Verification items for the finished model (mm, model axes). A direction names the side the tool comes from. Give positions to 0.01 mm unless a question says otherwise; leave off trailing zeros. Write each loop counter-clockwise with the first axis right and the second up, starting at its lowest first coordinate (ties: lowest second). Pieces come first, ordered by that corner, then holes. Notation, with made-up numbers: (2, 7) - (52, 7) arc R35 ccw to (52, 45) - close; hole circle Ø3 at (-22, 46.25). An arc over 180 degrees is marked (long way). Answer as a JSON object with one key per item and string values. Group by question number.
Item 1: Tool access check on faces 1 (the face through (-4.72, 3.48, -1.97)), 2 (the face through (-4.724, -3.448, -2.028)), 3 (the face through (-4.72, -3.48, 1.97)), 4 (the face through (0, 2.5, 2.5)), 5 (the face through (-4.724, 3.448, 2.028)). Record the directions out of +Z, -Z, +X, -X, +Y, -Y that give a thin tool (end or side, any length) a straight path to the whole face; none if there is none.
Item 2: Sectioned sample at A-A, the plane y = 0. Record the boundary of the cut face in (x, z).
Item 3: Scan lines: line 1 along X through (y, z) = (3.25, 1.5); line 2 along X through (y, z) = (-5, 2.5); line 3 along Y through (x, z) = (21, 2.5). Record each from-to range of solid material in increasing order. Write a range as [from, to].
Item 4: Go/stop test with flat-tipped pins: pin 1 (3 mm diameter, centred on x = 10, y = -3, fed in from +Z); pin 2 (5.5 mm diameter, centred on y = -0.5, z = -2.5, fed in from +X); pin 3 (1.5 mm diameter, centred on x = 17, z = 3, fed in from -Y); pin 4 (1.9 mm diameter, centred on x = -5.5, y = 0.5, fed in from -Z). Record where each tip stops, or that it passes through.
Item 5: Sectioned sample at B-B, the plane x = 29.5. Record the boundary of the cut face in (y, z).
Autodesk Inventor part; units mm, degrees
ref_plane "Work Plane1" through (10.95, 0, 0) normal (0, 0, -1) x (1, 0, 0)
ref_plane "YZ Plane" through (0, 0, 0) normal (1, 0, 0) x (0, 1, 0)
ref_plane "XZ Plane" through (0, 0, 0) normal (0, 1, 0) x (-1, 0, 0)
sketch "Schizzo1" plane through (0, 0, 0) normal (0, 0, 1) x (1, 0, 0)
  line L0 (-3.06, 0) -> (-3.06, 4.0996)
  line L1 (0, 5.7) -> (0, 3)
  line L2 (17, 3) -> (35, 3)
  line L3 (35, 3) -> (35, 0)
  line L4 (35, 0) -> (-3.06, 0)
  arc A0 (0, 5.7) -> (-2.0969, 6.1649) centre (-1.1, 5.7) ccw
  line L5 (0, -1.4013) -> (0, 8.4076)
  line L6 (-10.672, 0) -> (42.612, 0)
  line L7 (0, 3) -> (0.0001, 3)
  line L8 (0.0001, 3) -> (0.0001, 3)
  line L9 (0.0001, 3) -> (16.3865, 3)
  line L10 (16.3865, 3) -> (17, 3)
  line L11 (-3.06, 4.0996) -> (-2.0969, 6.1649)
  line L12 (0.0001, 3) -> (17, 3) construction
  line L13 (17, 3) -> (17, 0) construction
  dimension "d0" = 1.1
  dimension "d1" = 35
  dimension "d2" = 18
  dimension "d3" = 13.6
  dimension "d4" = 6
  dimension "d5" = 3.06
  dimension "d15" = 6
  dimension "d16" = 6
  dimension "d17" = 0.0001
  dimension "d18" = 0.6135
  dimension "d19" = 25
revolve "Corpo" add sketch "Schizzo1" angle 360 about axis through (35, 0, 0) along (-1, 0, 0)
sketch "Schizzo2" plane through (0, 0, 0) normal (1, 0, 0) x (0, 0, -1)
  line L0 (4, 2.3094) -> (4, -2.3094)
  line L1 (4, -2.3094) -> (0, -4.6188)
  line L2 (0, -4.6188) -> (-4, -2.3094)
  line L3 (-4, -2.3094) -> (-4, 2.3094)
  line L4 (-4, 2.3094) -> (0, 4.6188)
  line L5 (0, 4.6188) -> (4, 2.3094)
  point P0 (0, 0)
  point P1 (0, 0)
  dimension "d23" = 8
extrude "Testa" add sketch "Schizzo2" against normal blind 6.8
sketch "Schizzo3" plane through (0, 0, 0) normal (0, 0, 1) x (1, 0, 0)
  line L0 (-6.8, 3.8) -> (-6.8, 4.6188)
  line L1 (-6.8, 4.6188) -> (-6.3273, 4.6188)
  line L2 (-6.3273, 4.6188) -> (-6.8, 3.8)
  line L3 (-7.5964, 0) -> (-2.0215, 0)
  line L4 (-6.8, 4.6188) -> (-6.8, 2.3094)
  line L5 (-2.8179, 4.6188) -> (-6.8, 4.6188)
  point P0 (-6.8, 2.3094)
  dimension "d8" = 30
  dimension "d22" = 7.6
revolve "Smusso1" cut sketch "Schizzo3" angle 360 about axis through (-10, 0, 0) along (1, 0, 0)
thread "Filettatura"
chamfer "Smusso2" distance 0.6135 distance2 0.6135 1 edges at (35, -3, 0) measured on face at (35, -0.3546, -0.3912)
ref_plane "Work Plane1" through (10.95, 0, 0) normal (0, 0, -1) x (1, 0, 0)
equation "\"d0\" = PHH"
equation "\"d1\" = NLG"
equation "\"d2\" = GEL"
equation "\"d3\" = LADI"
equation "\"d4\" = GD"
equation "\"d5\" = 0.45 * KOH"
equation "\"d15\" = SD2"
equation "\"d16\" = BDM"
equation "\"d18\" = GAL"
equation "\"d19\" = KEWI"
equation "\"d23\" = SW"
equation "\"d6\" = KOH"
equation "\"d8\" = ANG1"
equation "\"d22\" = SW0"
equation "\"d10\" = GEL"
equation "\"d13\" = -0.5 * SPD + 0.5 * GD"
equation "\"d14\" = GUL"
equation "\"NLG\" = 35"
equation "\"GD\" = NND"
equation "\"BDM\" = NND"
equation "\"KOH\" = 6.8"
equation "\"GEL\" = 18"
equation "\"LADI\" = 13.6"
equation "\"SW\" = 8"
equation "\"PHH\" = RR"
equation "\"SW0\" = 7.6"
equation "\"SPD\" = NND - 1.2269 * PTC"
equation "\"SD2\" = NND"
equation "\"SD\" = 0"
equation "\"ANG1\" = 30deg"
equation "\"KEWI\" = 25deg"
equation "\"GAL\" = 0.61345 * PTC"
equation "\"GUL\" = 0.61345 * PTC"
equation "\"PTC\" = 1"
equation "\"THREADDIA\" = 6"
equation "\"E0\" = 1.155 * SW"
equation "\"TOA\" = 30deg"
equation "\"NND\" = 6"
equation "\"GD1\" = THREADDIA - 1.2269 * PTC"
equation "\"SDH\" = SW"
equation "\"KOH1\" = 2.9"
equation "\"RR\" = 1.1"
properties part number "ISO 4162 - M6 x 35" material "Acciaio inossidabile"
Geometry check:
{
 "1": {"face 1": "-Z, -X, +Y", "face 2": "-Z, -X, -Y", "face 3": "+Z, -X, -Y", "face 4": "+X", "face 5": "+Z, -X, +Y"},
 "2": {"outline": "(-6.8, -3.8) - (-6.68, -4) - (-3.06, -4) - (-3.06, -4.1) - (-2.1, -6.16) arc R1.1 ccw to (0, -5.7) - (0, -3) - (34.39, -3) - (35, -2.39) - (35, 2.39) - (34.39, 3) - (0, 3) - (0, 5.7) arc R1.1 ccw to (-2.1, 6.16) - (-3.06, 4.1) - (-3.06, 4) - (-6.68, 4) - (-6.8, 3.8) - close"},
 "3": {"line 1": "[-6.8, 0]", "line 2": "[-2.36, 0]", "line 3": "[-1.66, 1.66]"},
 "4": {"pin 1": "z = 2.6", "pin 2": "x = 35", "pin 3": "y = -1.98", "pin 4": "z = -4"},
 "5": {"outline": "circle Ø6 at (0, 0)"}
}
